Here's how the part is built. I have some questions about the finished solid (model axes, mm). A direction names the side the tool comes from. Coordinates: 2 decimals unless noted, no trailing zeros. Write each loop counter-clockwise with the first axis right and the second up, starting at its lowest first coordinate (ties: lowest second). Pieces come first, ordered by that corner, then holes. Notation, with made-up numbers: (-31.5, -8) - (6.5, -8) arc R17 cw to (6.5, 22) - close; hole circle Ø4 at (-33.5, 24). An arc over 180 degrees is marked (long way). Answer in a Markdown table with one row per item. Add a question column.
Item 1: Imagine slicing it at A-A (x = 17.5). Please give me the cut outline in (y, z), plus the area to 3 significant figures.
Item 2: We'd pull the mould along X, two halves only. Please class faces 4 (the face through (25.795, 1.521, -28.296)), 5 (the face through (-21.783, 1.479, 24.7)), 6 (the face through (10.3, 1.48, 5.81)), 7 (the face through (0, 3, 0)): +X half, -X half, draft (parallel to the pull), parting line (faces both ways), or undercut.
Item 3: Imagine slicing it at B-B (z = 23). Please give me the cut outline in (x, y), plus the area to 3 significant figures.
Item 4: Imagine slicing it at D-D (x = -22). Please give me the cut outline in (y, z).
Item 5: I'm going to push flat-ended pins straight in: pin 1 (1.5 mm diameter, centred on x = 12.5, y = 1, fed in from -Z); pin 2 (1 mm diameter, centred on y = 2, z = -13, fed in from -X). Where does each tip first touch, or does it pass through?
Item 6: If I drill on probe 1 along Z at (x, y) = (0, 1.65); probe 2 along X at (y, z) = (0.45, -8.5); probe 3 along X at (y, z) = (0.7, 2), over which ranges is the centre line in solid material (lowest first)? Write a range as from..to.
Item 7: Imagine slicing it at C-C (y = 1.85). Please give me the cut outline in (x, z).
Item 8: Which directions (+Z, -Z, +X, -X, +Y, -Y) give clear straight access to the entire face, cutting with the end or side of a thin tool? Please do faces 1 (the face through (-17.493, 1.521, 20.625)), 2 (the face through (22.083, 1.479, -25.039)), 3 (the face through (-10.378, 1.479, -5.973)).
from build123d import *

# Parameters (mm, degrees)
RESSALTO_EXTRUS_O1_DEPTH = 3
FILETE2_R                = 1
FILETE3_R                = 1
FILETE4_R                = 3
FILETE5_R                = 1
FILETE6_R                = 2
FILETE8_R                = 3
FILETE9_R                = 1
FILETE10_R               = 1
FILETE11_R               = 1
FILETE12_R               = 3


with BuildPart() as part:
    # Esboço1 → Ressalto-extrusão1 (new body)
    with BuildSketch(Plane(origin=(0, 0, 0), x_dir=(1, 0, 0), z_dir=(0, 1, 0))):
        with BuildLine():
            Line((-26.457513111, 0), (-26.457513111, -30))
            Line((-26.457513111, -30), (-17.5, -19.843134833))
            ThreePointArc((-17.5, -19.843134833), (10.885621722, -24.114378278), (26.457513111, 0))
            Line((26.457513111, 0), (26.457513111, 30))
            Line((26.457513111, 30), (17.5, 19.843134833))
            ThreePointArc((17.5, 19.843134833), (-10.885621722, 24.114378278), (-26.457513111, 0))
        make_face()
        with BuildLine():
            Line((5.009713089, -5.505167823), (3.030153969, -18.87502089))
            ThreePointArc((3.030153969, -18.87502089), (-16.899174829, -8.936785595), (-13.894779058, 13.129484439))
            Line((-13.894779058, 13.129484439), (-7.443392908, 0))
            ThreePointArc((-7.443392908, 0), (-3.009554378, -6.80783963), (5.009713089, -5.505167823))
        make_face(mode=Mode.SUBTRACT)
        with BuildLine():
            ThreePointArc((13.894779058, -13.129484439), (16.738722413, 9.233819289), (-3.694798692, 18.756244542))
            Line((-3.694798692, 18.756244542), (-5.200992817, 5.324825979))
            ThreePointArc((-5.200992817, 5.324825979), (2.888863526, 6.8599246), (7.443392908, 0))
            Line((7.443392908, 0), (13.894779058, -13.129484439))
        make_face(mode=Mode.SUBTRACT)
    extrude(amount=RESSALTO_EXTRUS_O1_DEPTH)

    # Filete2
    filete2_edges = [part.edges().sort_by_distance(p)[0] for p in [
        (26.457513111, 1.5, -30),
    ]]
    fillet(filete2_edges, radius=FILETE2_R)

    # Filete3
    filete3_edges = [part.edges().sort_by_distance(p)[0] for p in [
        (-26.457513111, 1.5, 30),
    ]]
    fillet(filete3_edges, radius=FILETE3_R)

    # Filete4
    filete4_edges = [part.edges().sort_by_distance(p)[0] for p in [
        (-5.200992817, 1.5, -5.324825979),
    ]]
    fillet(filete4_edges, radius=FILETE4_R)

    # Filete5
    filete5_edges = [part.edges().sort_by_distance(p)[0] for p in [
        (-3.694798692, 1.5, -18.756244542),
    ]]
    fillet(filete5_edges, radius=FILETE5_R)

    # Filete6
    filete6_edges = [part.edges().sort_by_distance(p)[0] for p in [
        (-17.5, 1.5, 19.843134833),
    ]]
    fillet(filete6_edges, radius=FILETE6_R)

    # Filete8
    filete8_edges = [part.edges().sort_by_distance(p)[0] for p in [
        (5.009713089, 1.5, 5.505167823),
    ]]
    fillet(filete8_edges, radius=FILETE8_R)

    # Filete9
    filete9_edges = [part.edges().sort_by_distance(p)[0] for p in [
        (3.030153969, 1.5, 18.87502089),
    ]]
    fillet(filete9_edges, radius=FILETE9_R)

    # Filete10
    filete10_edges = [part.edges().sort_by_distance(p)[0] for p in [
        (13.894779058, 1.5, 13.129484439),
    ]]
    fillet(filete10_edges, radius=FILETE10_R)

    # Filete11
    filete11_edges = [part.edges().sort_by_distance(p)[0] for p in [
        (-13.894779058, 1.5, -13.129484439),
    ]]
    fillet(filete11_edges, radius=FILETE11_R)

    # Filete12
    filete12_edges = [part.edges().sort_by_distance(p)[0] for p in [
        (17.5, 1.5, -19.843134833),
    ]]
    fillet(filete12_edges, radius=FILETE12_R)


solid = part.part
Here are the results:
| question | item | result |
|---|---|---|
| 1 | outline | (0, -20.99) - (3, -20.99) - (3, -7.69) - (0, -7.69) - close; (0, 7.69) - (3, 7.69) - (3, 19.84) - (0, 19.84) - close |
| 1 | area | 76.3 mm2 |
| 2 | face 4 | parting line |
| 2 | face 5 | undercut |
| 2 | face 6 | undercut |
| 2 | face 7 | draft |
| 3 | outline | (-26.46, 0) - (-20.28, 0) - (-20.28, 3) - (-26.46, 3) - close; (-13.08, 0) - (13.08, 0) - (13.08, 3) - (-13.08, 3) - close |
| 3 | area | 97.0 mm2 |
| 4 | outline | (0, -14.7) - (3, -14.7) - (3, 24.95) - (0, 24.95) - close |
| 5 | pin 1 | stops at z = -23.71 |
| 5 | pin 2 | stops at x = -23.32 |
| 6 | probe 1 | z = -26.46..-19.12, -7.44..7.44, 19.12..26.46 |
| 6 | probe 2 | x = -25.05..-17.12, -11.62..-4.01, 17.12..26.46 |
| 6 | probe 3 | x = -26.46..-19.01, -7.17..8.43, 19.01..26.38 |
| 7 | outline | (-26.46, 0) arc R26.46 ccw to (15.39, -21.52) arc R3 cw to (19.38, -21.98) - (24.71, -28.02) arc R1 ccw to (26.46, -27.35) - (26.46, 0) arc R26.46 ccw to (-16.06, 21.02) arc R2 cw to (-18.78, 21.29) - (-24.71, 28.02) arc R1 ccw to (-26.46, 27.35) - close; hole (-14.91, -11.97) arc R1 ccw to (-13.23, -11.78) - (-7.44, 0) arc R7.44 cw to (0.9, 7.39) arc R3 ccw to (4.22, 10.81) - (3.14, 18.14) arc R1 ccw to (2.27, 18.98) arc R19.12 ccw to start; hole (-4.6, -10.65) - (-3.78, -18.01) arc R1 ccw to (-2.94, -18.89) arc R19.12 ccw to (14.91, 11.97) arc R1 ccw to (13.23, 11.78) - (7.44, 0) arc R7.44 cw to (-1.16, -7.35) arc R3 ccw to start |
| 8 | face 1 | +Z, +Y, -Y |
| 8 | face 2 | -Z, +Y, -Y |
| 8 | face 3 | +Y, -Y |
